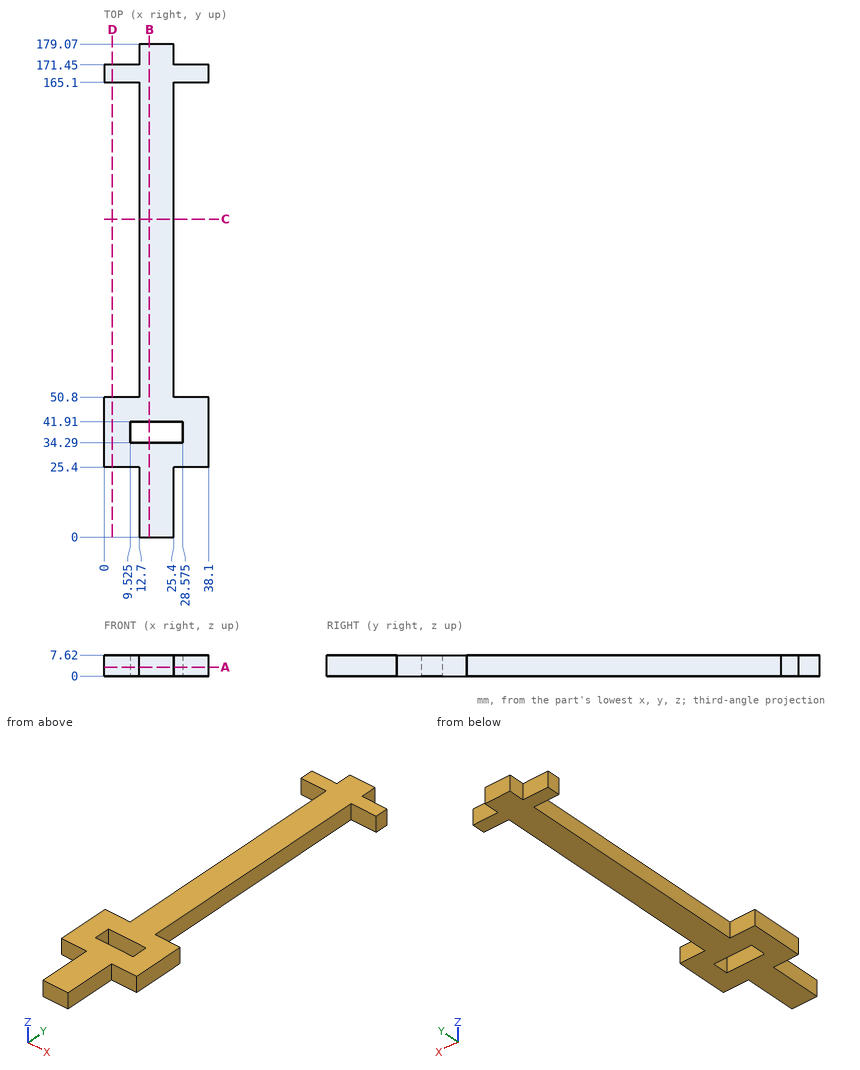
Design review of the part shown in the three views and the two pictorial views. Dimensions are in mm from the part's minimum x, y and z. Give positions to 0.01 mm unless a question says otherwise; leave off trailing zeros. Write each loop counter-clockwise with the first axis right and the second up, starting at its lowest first coordinate (ties: lowest second). Pieces come first, ordered by that corner, then holes. Notation, with made-up numbers: (85, -33) - (108, -33) arc R26 ccw to (108, 0) - close; hole circle Ø1 at (19.25, 78.5). An arc over 180 degrees is marked (long way). Return JSON: item names as keys, results as strings. Group by question number.
(1) We need section D-D, the plane x = 3. Give the boundary of the cut face in (y, z).
(2) We need section C-C, the plane y = 115.5. Give the boundary of the cut face in (x, z).
(3) We need section B-B, the plane x = 16.5. Give the boundary of the cut face in (y, z).
(4) We need section A-A, the plane z = 3.25. Give the boundary of the cut face in (x, y) (3 decimals).
(5) Insertion check: pin 1 (2.5 mm diameter, centred on y = 104, z = 5.5, fed in from +X); pin 2 (2.5 mm diameter, centred on x = 30, z = 3.5, fed in from -Y); pin 3 (2.5 mm diameter, centred on y = 175, z = 5.5, fed in from -X). Each pin has a flat end and moves straight along its axis. Give the tip position at first contact, or say it passes through.
(6) To check wall thickness, follow probe 1 along Y at (x, z) = (25.5, 7); probe 2 along Y at (x, z) = (35, 4.25); probe 3 along Y at (x, z) = (23.5, 6). State the ranges of each line that lie inside material, in increasing order.
Reported:
{
 "1": {"outline": "(25.4, 0) - (50.8, 0) - (50.8, 7.62) - (25.4, 7.62) - close; (165.1, 0) - (171.45, 0) - (171.45, 7.62) - (165.1, 7.62) - close"},
 "2": {"outline": "(12.7, 0) - (25.4, 0) - (25.4, 7.62) - (12.7, 7.62) - close"},
 "3": {"outline": "(0, 0) - (34.29, 0) - (34.29, 7.62) - (0, 7.62) - close; (41.91, 0) - (179.07, 0) - (179.07, 7.62) - (41.91, 7.62) - close"},
 "4": {"outline": "(0, 25.4) - (12.7, 25.4) - (12.7, 0) - (25.4, 0) - (25.4, 25.4) - (38.1, 25.4) - (38.1, 50.8) - (25.4, 50.8) - (25.4, 165.1) - (38.1, 165.1) - (38.1, 171.45) - (25.4, 171.45) - (25.4, 179.07) - (12.7, 179.07) - (12.7, 171.45) - (0, 171.45) - (0, 165.1) - (12.7, 165.1) - (12.7, 50.8) - (0, 50.8) - close; hole (9.525, 34.29) - (28.575, 34.29) - (28.575, 41.91) - (9.525, 41.91) - close"},
 "5": {"pin 1": "stops at x = 25.4", "pin 2": "stops at y = 25.4", "pin 3": "stops at x = 12.7"},
 "6": {"probe 1": "y = 25.4 to 34.29, 41.91 to 50.8, 165.1 to 171.45", "probe 2": "y = 25.4 to 50.8, 165.1 to 171.45", "probe 3": "y = 0 to 34.29, 41.91 to 179.07"}
}
